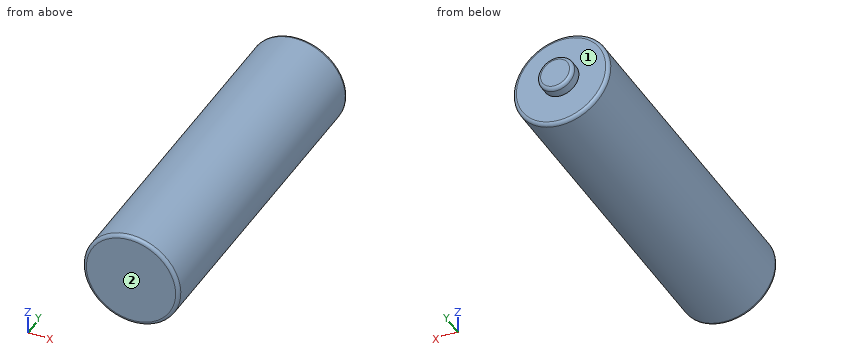
from build123d import *

# Parameters (mm, degrees)
SKETCH1_R           = 7.05
BOSS_EXTRUDE2_DEPTH = 48.25
SKETCH2_R           = 2.62
BOSS_EXTRUDE3_DEPTH = 1.71
FILLET1_R           = 0.5


with BuildPart() as part:
    # Sketch1 → Boss-Extrude2 (new body)
    with BuildSketch(Plane(origin=(0, 0, 0), x_dir=(1, 0, 0), z_dir=(0, 1, 0))):
        with Locations(Location((0, 0, 0), (0, 0, 270))):
            Circle(SKETCH1_R)
    extrude(amount=BOSS_EXTRUDE2_DEPTH)

    # Sketch2 → Boss-Extrude3 (add)
    with BuildSketch(Plane(origin=(0, 48.25, 0), x_dir=(1, 0, 0), z_dir=(0, 1, 0))):
        with Locations(Location((0, 0, 0), (0, 0, 270))):
            Circle(SKETCH2_R)
    extrude(amount=BOSS_EXTRUDE3_DEPTH)

    # Fillet1
    fillet1_edges = [part.edges().sort_by_distance(p)[0] for p in [
        (0, 0, -7.05),
        (0, 48.25, -7.05),
        (0, 49.96, -2.62),
    ]]
    fillet(fillet1_edges, radius=FILLET1_R)


solid = part.part
Design review of the part built by this model. Coordinates are the model's own, in mm. Face numbers are marked on the shaded views. A direction names the side the tool comes from. Round coordinates to 2 decimals unless told otherwise and drop trailing zeros. Write each loop counter-clockwise with the first axis right and the second up, starting at its lowest first coordinate (ties: lowest second). Pieces come first, ordered by that corner, then holes. Notation, with made-up numbers: (65, 23) - (111, 23) arc R30 cw to (111, 60) - close; hole circle Ø8 at (78, 12). An arc over 180 degrees is marked (long way). Return JSON: item names as keys, results as strings. Group by question number.
Item 1: We need section A-A on z = 0. Write out the cut boundary in (x, y).
Item 2: Machinability: for the marked faces 1 and 2, which of the approach directions +Z, -Z, +X, -X, +Y, -Y give a long, thin tool a straight path to every point of the face, cutting with its end or side? Answer none if there is none.
Item 3: For probe 1 along X at (y, z) = (30.5, -0.25); probe 2 along Y at (x, z) = (-2, -4); probe 3 along Z at (x, y) = (-4.5, 12.5), list the stretches that pass through material, from the lowest coordinate up. Write a range as [from, to].
Item 4: We need section B-B on y = 21. Write out the cut boundary in (x, z), and give its area (3 significant figures).
Item 5: Insertion check: P1, Ø5, axis at x = 5, y = 17, coming from the +Z side; P2, Ø4, axis at x = 4, z = 4.5, coming from the +Y side; P3, Ø2, axis at x = -1.5, y = 19.5, coming from the +Z side. Each pin has a flat end and moves straight along its axis. Give the tip position at first contact, or say it passes through.
Model answer:
{
 "1": {"outline": "(-7.05, 0.5) arc R0.5 ccw to (-6.55, 0) - (6.55, 0) arc R0.5 ccw to (7.05, 0.5) - (7.05, 47.75) arc R0.5 ccw to (6.55, 48.25) - (2.62, 48.25) - (2.62, 49.46) arc R0.5 ccw to (2.12, 49.96) - (-2.12, 49.96) arc R0.5 ccw to (-2.62, 49.46) - (-2.62, 48.25) - (-6.55, 48.25) arc R0.5 ccw to (-7.05, 47.75) - close"},
 "2": {"face 1": "+Y", "face 2": "+Z, -Z, +X, -X, -Y"},
 "3": {"probe 1": "x = [-7.05, 7.05]", "probe 2": "y = [0, 48.25]", "probe 3": "z = [-5.43, 5.43]"},
 "4": {"outline": "circle Ø14.1 at (0, 0)", "area": "156 mm²"},
 "5": {"P1": "stops at z = 6.59", "P2": "stops at y = 48.25", "P3": "stops at z = 7.03"}
}
